CAD build for the part. Positions are in the model's coordinates, mm. A direction names the side the tool comes from. Round coordinates to 2 decimals unless told otherwise and drop trailing zeros. Order: outer loops, then holes, each group sorted by start corner. A loop starts at its lowest first (then second) coordinate and runs counter-clockwise, first axis right, second up. Notation, with made-up numbers: (27.5, 64.5) - (69.5, 64.5) arc R18 cw to (69.5, 91.5) - close; hole circle Ø11 at (-12, 64.25). An arc over 180 degrees is marked (long way). Write item = value, one per line.
from build123d import *

# Parameters (mm, degrees)
SKETCH1_W               = 60
SKETCH1_H               = 145
BOSS_EXTRUDE1_DEPTH     = 10
BOSS_EXTRUDE2_DEPTH     = 45
SKETCH6_W               = 26.7
SKETCH6_H               = 24
CUT_EXTRUDE2_DEPTH      = 6
SKETCH8_R               = 1.15
CUT_EXTRUDE3_DEPTH      = 3
SKETCH9_W               = 60
SKETCH9_H               = 10
BOSS_EXTRUDE4_DEPTH     = 35
SKETCH12_W              = 6
SKETCH12_H              = 25
BOSS_EXTRUDE7_DEPTH     = 51
SKETCH13_R              = 8.05
SKETCH13_R_2            = 5.05
BOSS_EXTRUDE8_DEPTH     = 15
FILLET1_R               = 3
CUT_EXTRUDE4_REACH      = 160.348
CUT_EXTRUDE4_END_RADIUS = 8.05
SKETCH15_R              = 1.5
MIRROR1_START           = 9
MIRROR1_OUTLINE_R       = 8.05
MIRROR1_OUTLINE_R_2     = 5.05
MIRROR1_DEPTH           = 8.499999899
MIRROR1_START_2         = 20.499999166
MIRROR1_2_OUTLINE_R     = 8.05
MIRROR1_2_OUTLINE_R_2   = 5.05
MIRROR1_2_DEPTH         = 4.500000834
MIRROR1_START_3         = 17.499999899
MIRROR1_3_OUTLINE_R     = 8.05
MIRROR1_3_OUTLINE_R_2   = 5.05
MIRROR1_3_DEPTH         = 2.999999267
MIRROR1_START_4         = 18
MIRROR1_5_OUTLINE_R     = 1.5
MIRROR1_5_DEPTH         = 4.583753541
SKETCH17_W              = 10
SKETCH17_H              = 47
BOSS_EXTRUDE9_DEPTH     = 25
SKETCH18_W              = 10
SKETCH18_H              = 48
BOSS_EXTRUDE10_DEPTH    = 25
SKETCH19_R              = 2.5
CUT_EXTRUDE5_DEPTH      = 10
SKETCH20_W              = 60
SKETCH20_H              = 16
CUT_EXTRUDE6_DEPTH      = 10
CUT_EXTRUDE7_DEPTH      = 10
CUT_EXTRUDE8_DEPTH      = 10
FILLET2_R               = 20
CUT_EXTRUDE9_DEPTH      = 10
CUT_EXTRUDE10_DEPTH     = 101.361917618
CUT_EXTRUDE11_START     = -21
SKETCH26_W              = 30
SKETCH26_H              = 4
CUT_EXTRUDE11_DEPTH     = 21
SKETCH28_W              = 38
SKETCH28_H              = 30
CUT_EXTRUDE12_DEPTH     = 10
SKETCH29_R              = 1
SKETCH29_R_2            = 1.5
CUT_EXTRUDE13_DEPTH     = 12


with BuildPart() as part:
    # Sketch1 → Boss-Extrude1 (new body)
    with BuildSketch(Plane.XY):
        with Locations((30, 72.5)):
            Rectangle(SKETCH1_W, SKETCH1_H)
    extrude(amount=BOSS_EXTRUDE1_DEPTH)

    # Sketch2 → Boss-Extrude2 (add)
    with BuildSketch(Plane.XY.offset(10)):
        Polygon((4, 18), (49, 18), (49, 60.5), (34, 60.5), (34, 64.5), (55, 64.5), (55, 10), (4, 10), align=None)
    extrude(amount=BOSS_EXTRUDE2_DEPTH)

    # Sketch6 → Cut-Extrude2 (cut)
    with BuildSketch(Plane(origin=(55, 0, 0), x_dir=(0, 0, -1), z_dir=(1, 0, 0))):
        with Locations((-31.15, 39.2)):
            Rectangle(SKETCH6_W, SKETCH6_H)
    extrude(amount=-CUT_EXTRUDE2_DEPTH, mode=Mode.SUBTRACT)

    # Sketch8 → Cut-Extrude3 (cut)
    with BuildSketch(Plane(origin=(0, 64.5, 0), x_dir=(1, 0, 0), z_dir=(0, 1, 0))):
        with Locations(Location((49.25, -47.5, 0), (0, 0, 270))):
            Circle(SKETCH8_R)
        with Locations(Location((39.75, -47.5, 0), (0, 0, 270))):
            Circle(SKETCH8_R)
    extrude(amount=-CUT_EXTRUDE3_DEPTH, mode=Mode.SUBTRACT)

    # Sketch9 → Boss-Extrude4 (add)
    with BuildSketch(Plane.XZ):
        with Locations((30, 5)):
            Rectangle(SKETCH9_W, SKETCH9_H)
    extrude(amount=BOSS_EXTRUDE4_DEPTH)

    # Sketch12 → Boss-Extrude7 (add)
    with BuildSketch(Plane.ZY.offset(-4)):
        with Locations((49.02, -2.5)):
            Rectangle(SKETCH12_W, SKETCH12_H)
    extrude(amount=-BOSS_EXTRUDE7_DEPTH)

    # Sketch13 → Boss-Extrude8 (add)
    with BuildSketch(Plane.XY.offset(10)):
        with Locations(Location((27.39, 120.43, 0), (0, 0, 180))):
            Circle(SKETCH13_R)
        with Locations((27.39, 120.43)):
            Circle(SKETCH13_R_2, mode=Mode.SUBTRACT)
    extrude(amount=BOSS_EXTRUDE8_DEPTH)

    # Fillet1
    fillet1_edges = [part.edges().sort_by_distance(p)[0] for p in [
        (35.44, 120.43, 10),
    ]]
    fillet(fillet1_edges, radius=FILLET1_R)

    # Cut-Extrude4: up to this cylinder (the profile starts inside it)
    cut_extrude4_end = Plane(origin=(27.39, 120.43, 19), z_dir=(0, 0, -1)) * Cylinder(CUT_EXTRUDE4_END_RADIUS, 337.796, mode=Mode.PRIVATE)
    # Sketch15 → Cut-Extrude4 (cut, up to the surface)
    with BuildSketch(Plane.ZY.offset(-32), mode=Mode.PRIVATE) as cut_extrude4_sk1:
        with Locations(Location((19, 120.48, 0), (0, 0, 180))):
            Circle(SKETCH15_R)
    cut_extrude4_tool1 = extrude(cut_extrude4_sk1.sketch, amount=CUT_EXTRUDE4_REACH, mode=Mode.PRIVATE) & cut_extrude4_end
    add(cut_extrude4_tool1.solids().sort_by_distance((32, 120.48, 19))[0], mode=Mode.SUBTRACT)

    # Mirror1: read off the stored shape, not the designer's step
    # Mirror1 outline → Mirror1 (add)
    with BuildSketch(Plane.XY.offset(MIRROR1_START)):
        with Locations((27.39, 70.31)):
            Circle(MIRROR1_OUTLINE_R)
        with Locations((27.39, 70.31)):
            Circle(MIRROR1_OUTLINE_R_2, mode=Mode.SUBTRACT)
    extrude(amount=MIRROR1_DEPTH)



with BuildPart() as body_2:
    # Mirror1 2 outline → Mirror1 2 (new body)
    with BuildSketch(Plane.XY.offset(MIRROR1_START_2)):
        with Locations((27.39, 70.31)):
            Circle(MIRROR1_2_OUTLINE_R)
        with Locations((27.39, 70.31)):
            Circle(MIRROR1_2_OUTLINE_R_2, mode=Mode.SUBTRACT)
    extrude(amount=MIRROR1_2_DEPTH)


with BuildPart() as part_1:
    add(part.part)

    add(body_2.part)  # Mirror1 3 merges body 2
    # Mirror1 3 outline → Mirror1 3 (add)
    with BuildSketch(Plane.XY.offset(MIRROR1_START_3)):
        with Locations((27.39, 70.31)):
            Circle(MIRROR1_3_OUTLINE_R)
        with Locations((27.39, 70.31)):
            Circle(MIRROR1_3_OUTLINE_R_2, mode=Mode.SUBTRACT)
    extrude(amount=MIRROR1_3_DEPTH)

    # Mirror1 4 outline → Mirror1 4 (revolve)
    with BuildSketch(Plane(origin=(27.39, 70.31, 0), x_dir=(1, 0, 0), z_dir=(0, -1, 0))):
        with BuildLine():
            Line((8.05, 10), (11.05, 10))
            ThreePointArc((11.05, 10), (8.928679656, 10.878679656), (8.05, 13))
            Line((8.05, 13), (8.05, 10))
        make_face()
    revolve(axis=Axis((27.39, 70.31, 0), (0, 0, 1)))

    # Mirror1 5 outline → Mirror1 5 (cut)
    with BuildSketch(Plane.YZ.offset(MIRROR1_START_4)):
        with Locations((70.26, 19)):
            Circle(MIRROR1_5_OUTLINE_R)
    extrude(amount=MIRROR1_5_DEPTH, mode=Mode.SUBTRACT)

    # Sketch17 → Boss-Extrude9 (add)
    with BuildSketch(Plane(origin=(60, 0, 0), x_dir=(0, 0, -1), z_dir=(1, 0, 0))):
        with Locations((-5, 103.5)):
            Rectangle(SKETCH17_W, SKETCH17_H)
    extrude(amount=BOSS_EXTRUDE9_DEPTH)

    # Sketch18 → Boss-Extrude10 (add)
    with BuildSketch(Plane(origin=(60, 0, 0), x_dir=(0, 0, -1), z_dir=(1, 0, 0))):
        with Locations((-5, 5)):
            Rectangle(SKETCH18_W, SKETCH18_H)
    extrude(amount=BOSS_EXTRUDE10_DEPTH)

    # Sketch19 → Cut-Extrude5 (cut)
    with BuildSketch(Plane(origin=(0, 0, 0), x_dir=(-1, 0, 0), z_dir=(0, 0, -1))):
        with Locations((-73.238071341, 117.5)):
            Circle(SKETCH19_R)
        with Locations((-52.238071341, 117.5)):
            Circle(SKETCH19_R)
        with Locations((-52.238071341, 89.5)):
            Circle(SKETCH19_R)
        with Locations((-73.238071341, 89.5)):
            Circle(SKETCH19_R)
    cut_extrude5 = extrude(amount=-CUT_EXTRUDE5_DEPTH, mode=Mode.SUBTRACT)

    # Mirror2: Cut-Extrude5 across plane
    add(cut_extrude5.mirror(Plane.ZX.offset(54.95)), mode=Mode.SUBTRACT)

    # Sketch20 → Cut-Extrude6 (cut)
    with BuildSketch(Plane(origin=(0, 0, 0), x_dir=(-1, 0, 0), z_dir=(0, 0, -1))):
        with Locations((-30, -27)):
            Rectangle(SKETCH20_W, SKETCH20_H)
    extrude(amount=-CUT_EXTRUDE6_DEPTH, mode=Mode.SUBTRACT)

    # Sketch21 → Cut-Extrude7 (cut)
    with BuildSketch(Plane(origin=(0, 0, 0), x_dir=(-1, 0, 0), z_dir=(0, 0, -1))):
        with BuildLine():
            Line((-41.91493827, -19), (0, -19))
            Line((0, -19), (0, 9.855190418))
            add(Edge.make_bspline(
                [(0, 9.855190418), (-7.991882229, -11.003231013), (-38.248988904, 4.307186348), (-41.91493827, -19)],
                knots=[0, 0, 0, 0, 1, 1, 1, 1], degree=3))
        make_face()
    extrude(amount=-CUT_EXTRUDE7_DEPTH, mode=Mode.SUBTRACT)

    # Sketch22 → Cut-Extrude8 (cut)
    with BuildSketch(Plane.XY.offset(10)):
        with BuildLine():
            Line((14.869359674, 145), (0, 145))
            Line((0, 145), (0, 55.753772628))
            add(Edge.make_bspline(
                [(0, 55.753772628), (22.996880837, 81.13600087), (-6.640389726, 120.566568951), (14.869359674, 145)],
                knots=[0, 0, 0, 0, 1, 1, 1, 1], degree=3))
        make_face()
    extrude(amount=-CUT_EXTRUDE8_DEPTH, mode=Mode.SUBTRACT)

    # Fillet2
    fillet2_edges = [part_1.edges().sort_by_distance(p)[0] for p in [
        (0, 9.855190418, 5),
        (0, 55.753772628, 5),
        (14.869359674, 145, 5),
    ]]
    fillet(fillet2_edges, radius=FILLET2_R)

    # Sketch23 → Cut-Extrude9 (cut)
    with BuildSketch(Plane.XY.offset(10)):
        with BuildLine():
            Line((41.308294674, 145), (60, 145))
            Line((60, 145), (60, 127))
            add(Edge.make_bspline(
                [(60, 127), (54.009421291, 139.215727594), (41.308294674, 145)],
                knots=[0, 0, 0, 1, 1, 1], degree=2))
        make_face()
    extrude(amount=-CUT_EXTRUDE9_DEPTH, mode=Mode.SUBTRACT)

    # Sketch24 → Cut-Extrude10 (cut)
    with BuildSketch(Plane(origin=(55, 0, 0), x_dir=(0, 0, -1), z_dir=(1, 0, 0))):
        with BuildLine():
            Line((-46.65, 53.1), (-48.65, 53.1))
            ThreePointArc((-48.65, 53.1), (-50.2, 54.65), (-48.65, 56.2))
            Line((-48.65, 56.2), (-46.65, 56.2))
            ThreePointArc((-46.65, 56.2), (-45.1, 54.65), (-46.65, 53.1))
        make_face()
        with BuildLine():
            Line((-15.65, 53.1), (-17.65, 53.1))
            ThreePointArc((-17.65, 53.1), (-19.2, 54.65), (-17.65, 56.2))
            Line((-17.65, 56.2), (-15.65, 56.2))
            ThreePointArc((-15.65, 56.2), (-14.1, 54.65), (-15.65, 53.1))
        make_face()
        with BuildLine():
            Line((-15.65, 22.1), (-17.65, 22.1))
            ThreePointArc((-17.65, 22.1), (-19.2, 23.65), (-17.65, 25.2))
            Line((-17.65, 25.2), (-15.65, 25.2))
            ThreePointArc((-15.65, 25.2), (-14.1, 23.65), (-15.65, 22.1))
        make_face()
        with BuildLine():
            Line((-46.65, 22.1), (-48.65, 22.1))
            ThreePointArc((-48.65, 22.1), (-50.2, 23.65), (-48.65, 25.2))
            Line((-48.65, 25.2), (-46.65, 25.2))
            ThreePointArc((-46.65, 25.2), (-45.1, 23.65), (-46.65, 22.1))
        make_face()
    extrude(amount=-CUT_EXTRUDE10_DEPTH, mode=Mode.SUBTRACT)

    # Sketch26 → Cut-Extrude11 (cut)
    with BuildSketch(Plane.ZY.offset(-34).offset(CUT_EXTRUDE11_START)):
        with Locations((25, 62.5)):
            Rectangle(SKETCH26_W, SKETCH26_H)
    extrude(amount=CUT_EXTRUDE11_DEPTH, mode=Mode.SUBTRACT)

    # Sketch28 → Cut-Extrude12 (cut)
    with BuildSketch(Plane(origin=(0, 0, 0), x_dir=(-1, 0, 0), z_dir=(0, 0, -1))):
        with Locations((-19, 34.007303443)):
            Rectangle(SKETCH28_W, SKETCH28_H)
    extrude(amount=-CUT_EXTRUDE12_DEPTH, mode=Mode.SUBTRACT)

    # Sketch29 → Cut-Extrude13 (cut)
    with BuildSketch(Plane(origin=(0, 0, 46.02), x_dir=(-1, 0, 0), z_dir=(0, 0, -1))):
        with Locations((-11, -11)):
            Circle(SKETCH29_R)
        with Locations((-27, -3.5)):
            Circle(SKETCH29_R_2)
        with Locations((-11, 4)):
            Circle(SKETCH29_R)
        with Locations((-43, 4)):
            Circle(SKETCH29_R)
        with Locations((-43, -11)):
            Circle(SKETCH29_R)
    extrude(amount=-CUT_EXTRUDE13_DEPTH, mode=Mode.SUBTRACT)


solid = part_1.part
(1) Tool access for faces 1 (the cylindrical face through (52, 54.6, 19.2)), 2 (the cylindrical face through (20.98, 120.41, 20.5)), 3 (the flat face through (72, 29, 5)): list every direction of +Z, -Z, +X, -X, +Y, -Y with a clear straight run to the whole face (end or side of a thin tool).
Solved:
face_1 = +X, -X
face_2 = -X
face_3 = +Z, -Z, +X
(2) Probe line 1 along Y through (x, z) = (11, 50); line 2 along Y through (x, z) = (54.5, 43.5); line 3 along Y through (x, z) = (53, 38.5). List the from-to ranges inside material, lowest first.
Solved:
line_1 = -15 to -12, -10 to 3, 5 to 18
line_2 = 10 to 27.2, 51.2 to 64.5
line_3 = 10 to 27.2, 51.2 to 60.5
(3) Band-saw the part on B-B on z = 4. Count the separate pieces of the cut face and the enclosed holes in it, plus the area to 3 significant figures.
Solved:
separate_pieces = 1
enclosed_holes = 8
area = 9,380 mm²
(4) Pull direction Z, two halves, no side cores. Call faces 4 (the cylindrical face through (52, 23.6, 50.2)), 5 (the cylindrical face through (52.56, 91.98, 4.93)), 6 (the flat face through (30, 10, 28)): released by +Z, released by -Z, zero draft, split by the parting line, or undercut.
Solved:
face_4 = undercut
face_5 = zero draft
face_6 = undercut
(5) Drop flat-ended pins along their axis: pin 1 (1 mm diameter, centred on x = 16.5, z = 44.5, fed in from +Y); pin 2 (0.8 mm diameter, centred on x = 35, z = 10.5, fed in from -Y); pin 3 (17.5 mm diameter, centred on x = 25, y = 73.5, fed in from +Z). Give the stop position or say it passes through.
Solved:
pin_1 = 18
pin_2 = 10
pin_3 = 25
(6) Band-saw the part on A-A on z = 42. List the corners of the cut face in (x, y), plus the area to 3 significant figures.
Solved:
outline = (4, 10) - (55, 10) - (55, 27.2) - (49, 27.2) - (49, 18) - (4, 18) - close; (34, 60.5) - (49, 60.5) - (49, 51.2) - (55, 51.2) - (55, 64.5) - (34, 64.5) - close
area = 603 mm²
